Geometry check sheet. Reference: the model listing, model coordinates, mm. Face numbers are marked on the shaded views. A direction names the side the tool comes from. Round coordinates to 2 decimals unless told otherwise and drop trailing zeros. Loops run counter-clockwise (first coordinate to the right, second up) from the corner with the lowest first, then second, coordinate; pieces in that order, holes last. Notation, with made-up numbers: M 33.25,-21 L 71.25,-21 A24 cw 71.25,13 Z; hole C -27.75,-39 d2. An arc over 180 degrees is marked long. Write item = value, one per line.
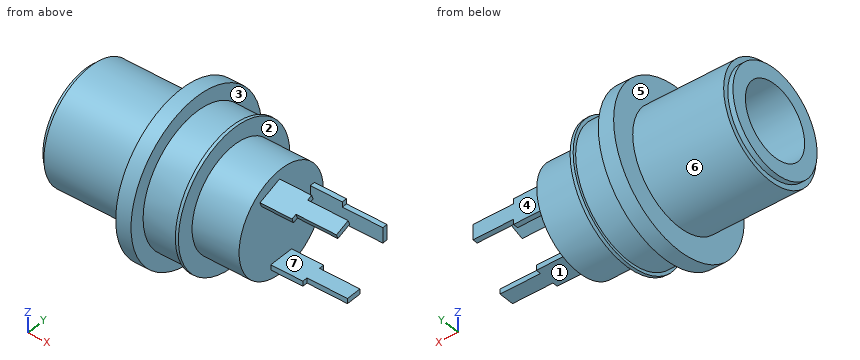
from build123d import *

# Parameters (mm, degrees)
SKETCH2_R           = 3.55625
CUT_EXTRUDE1_DEPTH  = 7.9
SKETCH3_W           = 2.5
SKETCH3_H           = 0.5
SKETCH3_W_2         = 0.5
SKETCH3_H_2         = 2.5
EXTRUDE_THIN1_DEPTH = 7.1
SKETCH4_W           = 0.5
SKETCH4_H           = 0.5
CUT_EXTRUDE3_DEPTH  = 3.96


with BuildPart() as part:
    # Sketch1 → Revolve1 (revolve)
    with BuildSketch(Plane.XY):
        Polygon((-19.2, 0), (-19.2, 5.05625), (-18.7, 5.05625), (-18.7, 5.55625), (-9.8, 5.55625), (-9.8, 7.85), (-8.3, 7.85), (-8.3, 6.4), (-4.9, 6.4), (-4.9, 6.7), (-4.6, 6.7), (-4.6, 5.05625), (0, 5.05625), (0, 0), align=None)
    revolve(axis=Axis((0, 0, 0), (-1, 0, 0)))

    # Sketch2 → Cut-Extrude1 (cut)
    with BuildSketch(Plane.ZY.offset(19.2)):
        with Locations(Location((0, 0, 0), (0, 0, 270))):
            Circle(SKETCH2_R)
    extrude(amount=-CUT_EXTRUDE1_DEPTH, mode=Mode.SUBTRACT)

    # Sketch3 → Extrude-Thin1 (add)
    with BuildSketch(Plane(origin=(0, 0, 0), x_dir=(0, 0, -1), z_dir=(1, 0, 0))):
        with Locations((0, 3.75)):
            Rectangle(SKETCH3_W, SKETCH3_H)
        with Locations((3.75, 0)):
            Rectangle(SKETCH3_W_2, SKETCH3_H_2)
        Polygon((-4.186295662, -0.193464797), (-3.331245304, -2.542696349), (-2.861398994, -2.371686278), (-3.716449352, -0.022454726), align=None)
    extrude(amount=EXTRUDE_THIN1_DEPTH)

    # Sketch4 → Cut-Extrude3 (cut)
    with BuildSketch(Plane(origin=(7.1, 0, 0), x_dir=(0, 0, -1), z_dir=(1, 0, 0))):
        with Locations((-1, 3.75)):
            Rectangle(SKETCH4_W, SKETCH4_H)
        with Locations((1, 3.75)):
            Rectangle(SKETCH4_W, SKETCH4_H)
        with Locations((3.75, 1)):
            Rectangle(SKETCH4_W, SKETCH4_H)
        with Locations((3.75, -1)):
            Rectangle(SKETCH4_W, SKETCH4_H)
        Polygon((-3.331245304, -2.542696349), (-2.861398994, -2.371686278), (-3.032409065, -1.901839967), (-3.502255376, -2.072850039), align=None)
        Polygon((-3.716449352, -0.022454726), (-4.186295662, -0.193464797), (-4.015285591, -0.663311108), (-3.54543928, -0.492301036), align=None)
    extrude(amount=-CUT_EXTRUDE3_DEPTH, mode=Mode.SUBTRACT)


solid = part.part
(1) Sectioned sample at C-C on y = 3. Record the cut outline in (x, z), then the cut area to 3 significant figures.
Result set:
outline = M -19.2,-4.07 L -18.7,-4.07 L -18.7,-4.68 L -9.8,-4.68 L -9.8,-7.25 L -8.3,-7.25 L -8.3,-5.65 L -4.9,-5.65 L -4.9,-5.99 L -4.6,-5.99 L -4.6,-4.07 L 0,-4.07 L 0,4.07 L -4.6,4.07 L -4.6,5.99 L -4.9,5.99 L -4.9,5.65 L -8.3,5.65 L -8.3,7.25 L -9.8,7.25 L -9.8,4.68 L -18.7,4.68 L -18.7,4.07 L -19.2,4.07 L -19.2,1.91 L -11.3,1.91 L -11.3,-1.91 L -19.2,-1.91 Z
area = 158 mm2
(2) Sectioned sample at D-D on x = -3. Record the cut outline in (y, z), then the cut area to 3 significant figures.
Result set:
outline = C 0,0 d10.11
area = 80.3 mm2
(3) Sectioned sample at B-B on x = -14.25. Record the cut outline in (y, z).
Result set:
outline = C 0,0 d11.11; hole C 0,0 d7.11
(4) Depth check by flat-ended pin: pin 1 Ø2 at (x, z) = (3.5, -0.5) entering from -Y; pin 2 Ø3 at (x, z) = (-1.5, 3.5) entering from +Y; pin 3 Ø1 at (y, z) = (4.5, 4) entering from -X. Enter the tip coordinate at first touch or a pass-through.
Result set:
pin_1 = 3.5
pin_2 = 4.64
pin_3 = -18.7
(5) Material ranges on line 1 along Z through (x, y) = (-13.75, 0); line 2 along X through (y, z) = (6, 2.5); line 3 along X through (y, z) = (3, 3.75), recorded low to high. Write a range as from..to.
Result set:
line_1 = -5.56..-3.56, 3.56..5.56
line_2 = -9.8..-8.3, -4.9..-4.6
line_3 = -19.2..0
(6) Release check for a two-part mould opening along Z. For the marked faces 5, 6 and 7 record: released by +Z, released by -Z, zero draft, split by the parting line, or undercut.
Result set:
face_5 = zero draft
face_6 = split by the parting line
face_7 = undercut
(7) Tool access check on the marked faces 1, 2, 3 and 4. Record the directions out of +Z, -Z, +X, -X, +Y, -Y that give a thin tool (end or side, any length) a straight path to the whole face; none if there is none.
Result set:
face_1 = -Z, +X, +Y, -Y
face_2 = +X
face_3 = none
face_4 = +Z, -Z, +X, +Y
